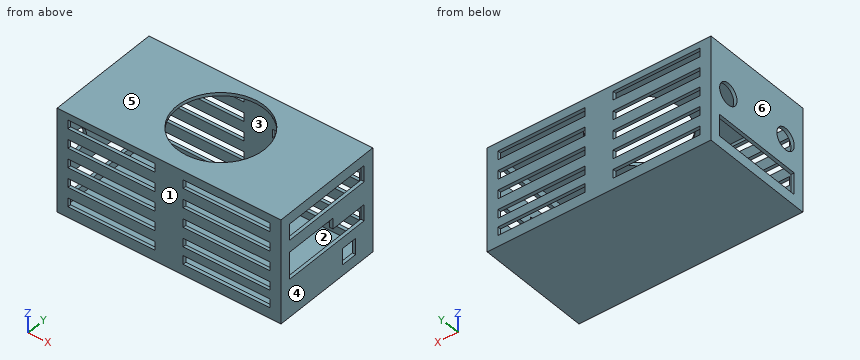
```python
from build123d import *

# Parameters (mm, degrees)
SKETCH1_W           = 206
SKETCH1_H           = 106
SKETCH1_W_2         = 200
SKETCH1_H_2         = 100
EXTRUDE_THIN1_DEPTH = 90
SKETCH2_W           = 206
SKETCH2_H           = 106
BOSS_EXTRUDE1_DEPTH = 3
SKETCH4_W           = 206
SKETCH4_H           = 106
BOSS_EXTRUDE2_DEPTH = 3
SKETCH5_R           = 40.274821778
CUT_EXTRUDE1_DEPTH  = 6
SKETCH6_W           = 80
SKETCH6_H           = 8
CUT_EXTRUDE2_DEPTH  = 150
SKETCH8_R           = 10
SKETCH8_W           = 20
SKETCH8_H           = 86
CUT_EXTRUDE3_DEPTH  = 10
SKETCH9_W           = 15
SKETCH9_H           = 15
SKETCH9_H_2         = 86
CUT_EXTRUDE4_DEPTH  = 10


with BuildPart() as part:
    # Sketch1 → Extrude-Thin1 (new body)
    with BuildSketch(Plane.XY):
        with Locations((25.793650794, -8.928571429)):
            Rectangle(SKETCH1_W, SKETCH1_H)
        with Locations((25.793650794, -8.928571429)):
            Rectangle(SKETCH1_W_2, SKETCH1_H_2, mode=Mode.SUBTRACT)
    extrude(amount=EXTRUDE_THIN1_DEPTH)

    # Sketch2 → Boss-Extrude1 (add)
    with BuildSketch(Plane(origin=(0, 0, 0), x_dir=(-1, 0, 0), z_dir=(0, 0, -1))):
        with Locations((-25.793650794, -8.928571429)):
            Rectangle(SKETCH2_W, SKETCH2_H)
    extrude(amount=BOSS_EXTRUDE1_DEPTH)

    # Sketch4 → Boss-Extrude2 (add)
    with BuildSketch(Plane.XY.offset(90)):
        with Locations((25.793650794, -8.928571429)):
            Rectangle(SKETCH4_W, SKETCH4_H)
    extrude(amount=BOSS_EXTRUDE2_DEPTH)

    # Sketch5 → Cut-Extrude1 (cut)
    with BuildSketch(Plane.XY.offset(93)):
        with Locations((28.793650794, -5.928571429)):
            Circle(SKETCH5_R)
    extrude(amount=-CUT_EXTRUDE1_DEPTH, mode=Mode.SUBTRACT)

    # Sketch6 → Cut-Extrude2 (cut)
    with BuildSketch(Plane(origin=(0, 44.071428571, 0), x_dir=(1, 0, 0), z_dir=(0, 1, 0))):
        with Locations((-27.206349206, -11)):
            Rectangle(SKETCH6_W, SKETCH6_H)
        with Locations((78.793650794, -11)):
            Rectangle(SKETCH6_W, SKETCH6_H)
        with Locations((78.793650794, -27.034238135)):
            Rectangle(SKETCH6_W, SKETCH6_H)
        with Locations((78.793650794, -45.034238135)):
            Rectangle(SKETCH6_W, SKETCH6_H)
        with Locations((78.793650794, -63.034238135)):
            Rectangle(SKETCH6_W, SKETCH6_H)
        with Locations((78.793650794, -81.034238135)):
            Rectangle(SKETCH6_W, SKETCH6_H)
        with Locations((-27.206349206, -29)):
            Rectangle(SKETCH6_W, SKETCH6_H)
        with Locations((-27.206349206, -47)):
            Rectangle(SKETCH6_W, SKETCH6_H)
        with Locations((-27.206349206, -65)):
            Rectangle(SKETCH6_W, SKETCH6_H)
        with Locations((-27.206349206, -83)):
            Rectangle(SKETCH6_W, SKETCH6_H)
    extrude(amount=-CUT_EXTRUDE2_DEPTH, mode=Mode.SUBTRACT)

    # Sketch8 → Cut-Extrude3 (cut)
    with BuildSketch(Plane.ZY.offset(77.206349206)):
        with Locations((52, 24.071428571)):
            Circle(SKETCH8_R)
        with Locations((52, -41.928571429)):
            Circle(SKETCH8_R)
        with Locations((17, -8.928571429)):
            Rectangle(SKETCH8_W, SKETCH8_H)
    extrude(amount=-CUT_EXTRUDE3_DEPTH, mode=Mode.SUBTRACT)

    # Sketch9 → Cut-Extrude4 (cut)
    with BuildSketch(Plane(origin=(128.793650794, 0, 0), x_dir=(0, 0, -1), z_dir=(1, 0, 0))):
        Polygon((-32, 34.071428571), (-32, -51.928571429), (-57, -51.928571429), (-57, -1.928571429), (-47, -1.928571429), (-47, 34.071428571), align=None)
        with Locations((-14.5, 16.571428571)):
            Rectangle(SKETCH9_W, SKETCH9_H)
        with Locations((-75.5, -8.928571429)):
            Rectangle(SKETCH9_W, SKETCH9_H_2)
    extrude(amount=-CUT_EXTRUDE4_DEPTH, mode=Mode.SUBTRACT)


solid = part.part
```
Geometry check sheet. Reference: the model listing, model coordinates, mm. Face numbers are marked on the shaded views. A direction names the side the tool comes from. Give positions to 0.01 mm unless a question says otherwise; leave off trailing zeros. Order: outer loops, then holes, each group sorted by start corner. A loop starts at its lowest first (then second) coordinate and runs counter-clockwise, first axis right, second up. Notation, with made-up numbers: (-31, 53.25) - (10, 53.25) arc R29 cw to (10, 88.25) - close; hole circle Ø6 at (30.5, 47.5). An arc over 180 degrees is marked (long way). Write item = value, one per line. Start each with the question number.
1) Scan lines: L1, parallel to Y at x = -75, z = 52; L2, parallel to Y at x = 39.5, z = 86.5; L3, parallel to Z at x = 80, y = -17. Record each from-to range of solid material in increasing order.
2) Section check D-D (x = -24). Count the separate pieces of the cut face and the enclosed holes in it, then the cut area to 3 significant figures.
3) Section check B-B (y = -38.5). Enter the section's corners in (x, z), then the cut area to 3 significant figures.
4) Access from +Z, -Z, +X, -X, +Y, -Y to the whole of each face (thin tool, end or side, straight path). Record for the marked faces 1 and 2.
5) Gauge pin test, flat end, axial feed: pin 1 Ø1 at (y, z) = (-28, 33.5) entering from +X. Record the tip position at first contact, or that the pin passes through.
6) Section check C-C (z = 37). Enter the section's corners in (x, y).
7) Draft check along X on the marked faces 3, 4, 5 and 6. Enter one of: released by +X, released by -X, zero draft, split by the parting line, or undercut.
8) Section check A-A (z = 54). Enter the section's corners in (x, y), then the cut area to 3 significant figures.
Geometry check:
q1.L1 = -61.93 to -51.93, -31.93 to 14.07, 34.07 to 44.07
q1.L2 = -61.93 to -58.93, 41.07 to 44.07
q1.L3 = -3 to 0, 90 to 93
q2.separate_pieces = 10
q2.enclosed_holes = 0
q2.area = 936 mm2
q3.outline = (-77.21, -3) - (128.79, -3) - (128.79, 32) - (125.79, 32) - (125.79, 0) - (-74.21, 0) - (-74.21, 7) - (-77.21, 7) - close; (-77.21, 27) - (-74.21, 27) - (-74.21, 42.61) - (-77.21, 42.61) - close; (-77.21, 61.39) - (-74.21, 61.39) - (-74.21, 90) - (5.1, 90) - (5.1, 93) - (-77.21, 93) - close; (52.48, 90) - (125.79, 90) - (125.79, 83) - (128.79, 83) - (128.79, 93) - (52.48, 93) - close; (125.79, 57) - (128.79, 57) - (128.79, 68) - (125.79, 68) - close
q3.area = 1,400 mm2
q4.face_1 = +Z, -Z, +X, -X, -Y
q4.face_2 = none
q5.pin_1 = -74.21
q6.outline = (-77.21, -61.93) - (128.79, -61.93) - (128.79, -51.93) - (125.79, -51.93) - (125.79, -58.93) - (-74.21, -58.93) - (-74.21, 41.07) - (125.79, 41.07) - (125.79, 34.07) - (128.79, 34.07) - (128.79, 44.07) - (-77.21, 44.07) - close
q7.face_3 = undercut
q7.face_4 = released by +X
q7.face_5 = zero draft
q7.face_6 = released by -X
q8.outline = (-77.21, -61.93) - (128.79, -61.93) - (128.79, -51.93) - (125.79, -51.93) - (125.79, -58.93) - (-74.21, -58.93) - (-74.21, -51.73) - (-77.21, -51.73) - close; (-77.21, -32.13) - (-74.21, -32.13) - (-74.21, 14.27) - (-77.21, 14.27) - close; (-77.21, 33.87) - (-74.21, 33.87) - (-74.21, 41.07) - (125.79, 41.07) - (125.79, -1.93) - (128.79, -1.93) - (128.79, 44.07) - (-77.21, 44.07) - close
q8.area = 1,570 mm2
